Input: part model. Units: mm. Frame: model coordinates. Round coordinates to 2 decimals unless told otherwise and drop trailing zeros. Loops run counter-clockwise (first coordinate to the right, second up) from the corner with the lowest first, then second, coordinate; pieces in that order, holes last.
1) Section D-D, the plane x = 38.1. Return loops of the section in (y, z) (1 decimal).
2) Section C-C, the plane x = 63.5. Return loops of the section in (y, z) (3 decimals).
3) Section A-A, the plane y = 1. State how many separate pieces and enclosed holes the cut face has, and give its area (3 significant figures).
4) Ray query, line 1 along Z through (x, y) = (63.5, 0.8) (3 decimals); line 2 along Z through (x, y) = (11.5, 1.5); line 3 along Z through (x, y) = (40, 0.2). Return the intervals inside material, ascending.
5) Section B-B, the plane z = -12.7. Return loops of the section in (x, y) (3 decimals).
Autodesk Inventor part; units mm, degrees
ref_plane "YZ Plane" through (0, 0, 0) normal (1, 0, 0) x (0, 1, 0)
ref_plane "XZ Plane" through (0, 0, 0) normal (0, 1, 0) x (-1, 0, 0)
ref_plane "XY Plane" through (0, 0, 0) normal (0, 0, 1) x (1, 0, 0)
sketch "Sketch1" plane through (0, 0, 0) normal (0, 1, 0) x (-1, 0, 0)
  line L0 (0, 0) -> (-76.2, 0)
  line L1 (-76.2, 0) -> (-76.2, -215.9)
  line L2 (-76.2, -215.9) -> (0, -215.9)
  line L3 (0, -215.9) -> (0, 0)
  dimension "d0" = 76.2
  dimension "d1" = 215.9
extrude "Extrusion1" add sketch "Sketch1" along normal blind 3.175
sketch "Sketch2" plane through (0, 3.175, 0) normal (0, 1, 0) x (1, 0, 0)
  line L0 (0, 0) -> (76.2, 0)
  line L1 (0, 215.9) -> (0, 0)
  circle A0 centre (12.7, 107.95) radius 2.54
  circle A1 centre (63.5, 107.95) radius 2.54
  circle A2 centre (38.1, 107.95) radius 7.9375
  dimension "d4" = 107.95
  dimension "d5" = 38.1
  dimension "d6" = 25.4
  dimension "d7" = 25.4
  dimension "d8" = 107.95
  dimension "d9" = 107.95
  dimension "d10" = 5.08
  dimension "d11" = 5.08
  dimension "d12" = 15.875
extrude "Extrusion2" cut sketch "Sketch2" against normal blind 25.4
sketch "Sketch3" plane through (0, 3.175, 0) normal (0, 1, 0) x (1, 0, 0)
  line L0 (0, 0) -> (76.2, 0)
  line L1 (76.2, 0) -> (76.2, 215.9)
  line L2 (76.2, 215.9) -> (0, 215.9)
  line L3 (0, 215.9) -> (0, 0)
  point P0 (12.7, 12.7)
  point P1 (63.5, 12.7)
  point P2 (63.5, 203.2)
  point P3 (12.7, 203.2)
  dimension "d15" = 12.7
  dimension "d16" = 12.7
  dimension "d17" = 12.7
  dimension "d18" = 12.7
  dimension "d19" = 12.7
  dimension "d20" = 12.7
  dimension "d21" = 12.7
  dimension "d22" = 12.7
hole "Hole1" at (12.7, 3.175, -12.7) at (63.5, 3.175, -12.7) at (63.5, 3.175, -203.2) at (12.7, 3.175, -203.2) direction (0, -1, 0) diameter 6.35 end through all
properties part number "motor support plate" material "Aluminum 6061"
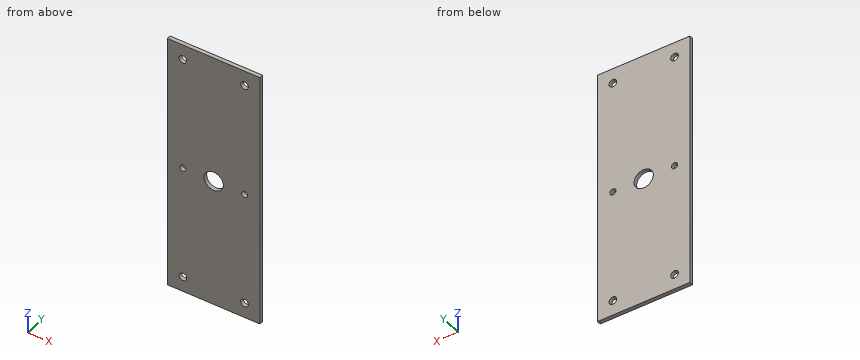
Final values:
1. outline: (0, -215.9) - (3.2, -215.9) - (3.2, -115.9) - (0, -115.9) - close; (0, -100) - (3.2, -100) - (3.2, 0) - (0, 0) - close
2. outline: (0, -215.9) - (3.175, -215.9) - (3.175, -206.375) - (0, -206.375) - close; (0, -200.025) - (3.175, -200.025) - (3.175, -110.49) - (0, -110.49) - close; (0, -105.41) - (3.175, -105.41) - (3.175, -15.875) - (0, -15.875) - close; (0, -9.525) - (3.175, -9.525) - (3.175, 0) - (0, 0) - close
3. separate pieces: 1
3. enclosed holes: 7
3. area: 16,100 mm2
4. line 1: z = -215.9 to -206.375, -200.025 to -110.49, -105.41 to -15.875, -9.525 to 0
4. line 2: z = -215.9 to -206.14, -200.26 to -110.19, -105.71 to -15.64, -9.76 to 0
4. line 3: z = -215.9 to -115.66, -100.24 to 0
5. outline: (0, 0) - (9.525, 0) - (9.525, 3.175) - (0, 3.175) - close; (15.875, 0) - (60.325, 0) - (60.325, 3.175) - (15.875, 3.175) - close; (66.675, 0) - (76.2, 0) - (76.2, 3.175) - (66.675, 3.175) - close
